```python
from build123d import *

# Parameters (mm, degrees)
F1_DEPTH        = 10
F2_R            = 21.75
F2_R_2          = 18.75
F3_DEPTH        = 20
F4_DEPTH        = 8
F7_DEPTH        = 3
F8_W            = 6
F8_H            = 40
F9_DEPTH        = 5
F11_D           = 2.2
F11_CSINK_D     = 5.1
F11_CSINK_ANGLE = 90


# Not quite as in the source:
# - a pattern or mirror of a feature is missing from the dataset's text; its kind, count and spacing are read off the source's solid


with BuildPart() as f1:
    # F0 (on Top) → F1 (new body)
    with BuildSketch(Plane.XY):
        Polygon((6.8993357168, 11.95), (-6.8993357168, 11.95), (-13.7986714336, 0), (-6.8993357168, -11.95), (6.8993357168, -11.95), (13.7986714336, 0), align=None)
        Polygon((-10.3345698185, 0), (-5.1672849092, 8.95), (5.1672849092, 8.95), (10.3345698185, 0), (5.1672849092, -8.95), (-5.1672849092, -8.95), align=None, mode=Mode.SUBTRACT)
    extrude(amount=F1_DEPTH)



with BuildPart() as f3:
    # F2 (on face) → F3 (new body)
    with BuildSketch(Plane.XY.offset(10)):
        Circle(F2_R)
        Circle(F2_R_2, mode=Mode.SUBTRACT)
    extrude(amount=-F3_DEPTH)


with BuildPart() as f4:
    # F2 (on face) → F4 (new body)
    with BuildSketch(Plane.XY.offset(10)):
        Circle(F2_R)
        Circle(F2_R_2, mode=Mode.SUBTRACT)
        Circle(F2_R_2)
        Polygon((6.8993357168, 11.95), (13.7986714336, 0), (6.8993357168, -11.95), (-6.8993357168, -11.95), (-13.7986714336, 0), (-6.8993357168, 11.95), align=None, mode=Mode.SUBTRACT)
        Polygon((6.8993357168, -11.95), (13.7986714336, 0), (6.8993357168, 11.95), (-6.8993357168, 11.95), (-13.7986714336, 0), (-6.8993357168, -11.95), align=None)
        Polygon((5.1672849092, -8.95), (-5.1672849092, -8.95), (-10.3345698185, 0), (-5.1672849092, 8.95), (5.1672849092, 8.95), (10.3345698185, 0), align=None, mode=Mode.SUBTRACT)
        Polygon((-10.3345698185, 0), (-5.1672849092, -8.95), (5.1672849092, -8.95), (10.3345698185, 0), (5.1672849092, 8.95), (-5.1672849092, 8.95), align=None)
    extrude(amount=F4_DEPTH)


with BuildPart() as f1_1:
    add(f1.part)

    add(f3.part)  # F7 merges F3

    add(f4.part)  # F7 merges F4
    # F6 (on face) → F7 (join)
    with BuildSketch(Plane(origin=(5.3550892957, 3.0917622464, -5.9713601914), x_dir=(0.7822484827, -0.2864336826, 0.5532115841), z_dir=(0.622966541, 0.3596699002, -0.6946583705))):
        Polygon((7.5026214932, -3.9601203317), (5.2654806886, -6.6518114397), (15.9953805493, -15.5697354674), (18.2325213539, -12.8780443594), align=None)
    f7 = extrude(amount=-F7_DEPTH)

    # F7_copies: F7 across plane
    add(f7.mirror(Plane(origin=(0, 0, 0), x_dir=(0, 0, -1), z_dir=(0, -1, 0))))

    # F7_copies1: F7 across plane
    add(f7.mirror(Plane(origin=(0, 0, 0), x_dir=(0, 0, -1), z_dir=(-1, 0, 0))))

    # F7_copies2: F7 across plane
    add(f7.mirror(Plane(origin=(0, 0, 0), x_dir=(0.5, -0.8660254038, 0), z_dir=(-0.8660254038, -0.5, 0))))

    # F8 (on face) → F9 (cut)
    with BuildSketch(Plane.XY.offset(18)):
        Rectangle(F8_W, F8_H)
    extrude(amount=-F9_DEPTH, mode=Mode.SUBTRACT)

    # F11 (through all)
    with Locations(Plane(origin=(0, 0, 10), x_dir=(1, 0, 0), z_dir=(0, 0, -1))):
        with Locations((0, 15), (0, -15)):
            CounterSinkHole(F11_D / 2, F11_CSINK_D / 2, counter_sink_angle=F11_CSINK_ANGLE)


solid = f1_1.part
```
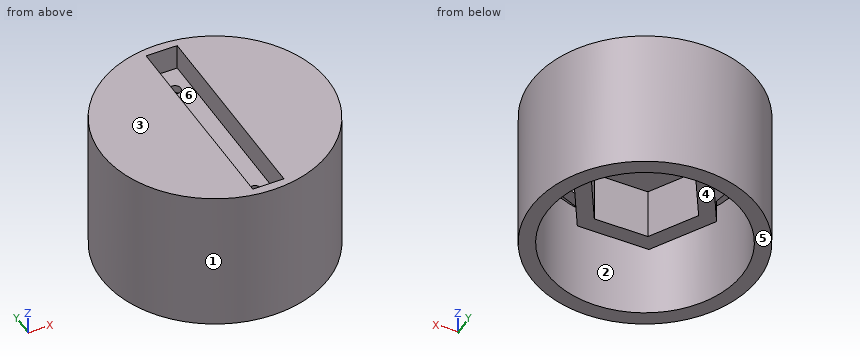
Verification items for the finished model (mm, model axes). Face numbers are marked on the shaded views. A direction names the side the tool comes from. Round coordinates to 2 decimals unless told otherwise and drop trailing zeros. Order: outer loops, then holes, each group sorted by start corner. A loop starts at its lowest first (then second) coordinate and runs counter-clockwise, first axis right, second up. Notation, with made-up numbers: (70, 50) - (108, 50) arc R23 ccw to (108, 79) - close; hole circle Ø10 at (69, -32.75). An arc over 180 degrees is marked (long way). Use CSV: the item, a comma, the result in double quotes. Start each with the question number.
1) Section check A-A, the plane y = 15. Record the cut outline in (x, z).
2) Access from +Z, -Z, +X, -X, +Y, -Y to the whole of each face (thin tool, end or side, straight path). Record for the marked faces 4, 5 and 6.
3) Go/stop test with flat-tipped pins: P1, Ø6, axis at y = 15, z = 6, coming from the +X side; P2, Ø19.5, axis at x = -1.5, y = 1.5, coming from the -Z side; P3, Ø2.5, axis at x = 0, y = 15, coming from the +Z side; P4, Ø8, axis at y = -2.5, z = 11.5, coming from the +X side. Record where each tip stops, or that it passes through.
4) Section check B-B, the plane x = 0. State how many separate pieces and enclosed holes the cut face has, plus the area to 3 significant figures.
5) Thickness scan on L1, parallel to Y at x = 0, z = 2.25; L2, parallel to Y at x = 0, z = 12.1; L3, parallel to Y at x = 7, z = 7. Record the ranges inside material, lowest first.
6) Section check C-C, the plane z = 14.25. Record the cut outline in (x, y).
7) Mould release check, pull along Y, two halves, no side actions. Record for the marked faces 1, 2 and 3: +Y half, -Y half, draft (parallel to the pull), parting line (faces both ways), or undercut.
Answers:
1,outline,"(-15.75, -10) - (-11.25, -10) - (-11.25, 10) - (-2.55, 10) - (-1.1, 11.45) - (-1.1, 13) - (-3, 13) - (-3, 18) - (-15.75, 18) - close; (1.1, 11.45) - (2.55, 10) - (11.25, 10) - (11.25, -10) - (15.75, -10) - (15.75, 18) - (3, 18) - (3, 13) - (1.1, 13) - close"
2,face 4,"-Z"
2,face 5,"-Z, +X, -X, +Y, -Y"
2,face 6,"+Z"
3,P1,"stops at x = 18.14"
3,P2,"stops at z = 0"
3,P3,"stops at z = 13"
3,P4,"stops at x = 21.75"
4,separate pieces,"3"
4,enclosed holes,"0"
4,area,"311 mm²"
5,L1,"y = -21.75 to -18.75, -11.95 to -8.95, 8.95 to 11.95, 18.75 to 21.75"
5,L2,"y = -21.75 to -16.1, -13.9 to 13.9, 16.1 to 21.75"
5,L3,"y = -20.59 to -17.39, -11.78 to -5.78, 5.78 to 11.78, 17.39 to 20.59"
6,outline,"circle Ø43.5 at (0, 0); hole (-3, -20) - (3, -20) - (3, 20) - (-3, 20) - close"
7,face 1,"parting line"
7,face 2,"undercut"
7,face 3,"draft"
